Check sheet for the modelled part. Datum: model origin and axes. Units: mm. A direction names the side the tool comes from. Round coordinates to 2 decimals unless told otherwise and drop trailing zeros. Write each loop counter-clockwise with the first axis right and the second up, starting at its lowest first coordinate (ties: lowest second). Pieces come first, ordered by that corner, then holes.
Autodesk Inventor part; units mm, degrees
ref_plane "YZ Plane" through (0, 0, 0) normal (1, 0, 0) x (0, 1, 0)
ref_plane "XZ Plane" through (0, 0, 0) normal (0, 1, 0) x (-1, 0, 0)
ref_plane "XY Plane" through (0, 0, 0) normal (0, 0, 1) x (1, 0, 0)
sketch "Sketch1" plane through (0, 0, 0) normal (0, 1, 0) x (-1, 0, 0)
  line L0 (0, 0) -> (42, 0)
  line L1 (42, 0) -> (42, -42)
  line L2 (42, -42) -> (0, -42)
  line L3 (0, -42) -> (0, 0)
  line L4 (42, -21) -> (42, -5.25)
  line L5 (21, -5.25) -> (36.75, -5.25)
  line L6 (36.75, -5.25) -> (5.25, -5.25)
  line L7 (5.25, -5.25) -> (5.25, -36.75)
  line L8 (5.25, -36.75) -> (36.75, -36.75)
  line L9 (36.75, -36.75) -> (36.75, -5.25)
  circle A0 centre (36.75, -5.25) radius 1.5
  circle A1 centre (36.75, -36.75) radius 1.5
  circle A2 centre (5.25, -36.75) radius 1.5
  circle A3 centre (5.25, -5.25) radius 1.5
  dimension "d6" = 3
  dimension "d7" = 3
  dimension "d8" = 3
  dimension "d9" = 3
extrude "Extrusion1" add sketch "Sketch1" along normal blind 43 contours L0 L1 L2 L3 | L5 A0 L9 A1 L8 A2 L7 A3 L6
sketch "Sketch2" plane through (0, 43, 0) normal (0, 1, 0) x (1, 0, 0)
  circle A0 centre (-21, 21) radius 11
  circle A1 centre (-21, 21) radius 2.5
  point P0 (0, 0)
  dimension "d12" = 22
  dimension "d15" = 5
extrude "Extrusion2" add sketch "Sketch2" along normal blind 3 contours A0 | A1
extrude "Extrusion3" add sketch "Sketch2" along normal blind 25 contours A1
sketch "Sketch3" plane through (0, 0, 0) normal (1, 0, 0) x (0, 0, -1)
  line L0 (42, 0) -> (0, 0)
  line L1 (21, 0) -> (28.5, 0)
  line L2 (28.5, 0) -> (13.5, 0)
  line L3 (13.5, 0) -> (13.5, 12)
  line L4 (13.5, 12) -> (28.5, 12)
  line L5 (28.5, 12) -> (28.5, 0)
  dimension "d18" = 7.5
  dimension "d19" = 15
  dimension "d20" = 12
extrude "Extrusion4" add sketch "Sketch3" along normal blind 8
fillet "Fillet1" radius 4 4 edges at (0, 21.5, 0) (0, 21.5, -42) (-42, 21.5, 0) (-42, 21.5, -42)
properties part number "stepperMotor"
1. Sectioned sample at C-C, the plane x = -36.75. Enter the section's corners in (y, z), plus the area to 3 significant figures.
2. Sectioned sample at A-A, the plane z = -36.75. Enter the section's corners in (x, y).
3. Sectioned sample at B-B, the plane y = 19. Enter the section's corners in (x, z), plus the area to 3 significant figures.
4. Release check for a two-part mould opening along X. For faces 4 (the flat face through (4, 6, -28.5)), 5 (the cylindrical face through (-4.925, 21.199, -35.286)), 6 (the flat face through (-42, 21, -21)), 7 (the cylindrical face through (-35.56, 21.2, -35.84)) record: released by +X, released by -X, zero draft, split by the parting line, or undercut.
5. Sectioned sample at D-D, the plane x = -21. Enter the section's corners in (y, z).
6. Go/stop test with flat-tipped pins: pin 1 (17 mm diameter, centred on y = 16, z = -26.5, fed in from +X); pin 2 (4 mm diameter, centred on x = 3, y = 7, fed in from +Z); pin 3 (2 mm diameter, centred on x = -3.5, z = -32, fed in from +Y); pin 4 (8 mm diameter, centred on y = 24, z = -23.5, fed in from +X). Record where each tip stops, or that it passes through.
7. Scan lines: line 1 along Z through (x, y) = (-5.25, 14); line 2 along X through (y, z) = (8, -6). Record each from-to range of solid material in increasing order.
8. Set-up check for faces 1 (the cylindrical face through (-15.924, 44.479, -30.759)), 2 (the flat face through (4, 12, -21)), 3 (the flat face through (-21, 21, -42)): record each of +Z, -Z, +X, -X, +Y, -Y from which the full face is reachable in a straight line by a thin tool's end or side.
Computed values:
1. outline: (0, -42) - (43, -42) - (43, -38.25) - (0, -38.25) - close; (0, -35.25) - (43, -35.25) - (43, -6.75) - (0, -6.75) - close; (0, -3.75) - (43, -3.75) - (43, 0) - (0, 0) - close
1. area: 1,550 mm2
2. outline: (-42, 0) - (-38.25, 0) - (-38.25, 43) - (-42, 43) - close; (-35.25, 0) - (-6.75, 0) - (-6.75, 43) - (-35.25, 43) - close; (-3.75, 0) - (0, 0) - (0, 43) - (-3.75, 43) - close
3. outline: (-42, -38) arc R4 ccw to (-38, -42) - (-4, -42) arc R4 ccw to (0, -38) - (0, -4) arc R4 ccw to (-4, 0) - (-38, 0) arc R4 ccw to (-42, -4) - close; hole circle Ø3 at (-36.75, -36.75); hole circle Ø3 at (-36.75, -5.25); hole circle Ø3 at (-5.25, -36.75); hole circle Ø3 at (-5.25, -5.25)
3. area: 1,720 mm2
4. face 4: zero draft
4. face 5: undercut
4. face 6: released by -X
4. face 7: undercut
5. outline: (0, -42) - (43, -42) - (43, -32) - (46, -32) - (46, -23.5) - (68, -23.5) - (68, -18.5) - (46, -18.5) - (46, -10) - (43, -10) - (43, 0) - (0, 0) - close
6. pin 1: stops at x = 8
6. pin 2: stops at z = -13.5
6. pin 3: stops at y = 43
6. pin 4: stops at x = 0
7. line 1: z = -42 to -38.25, -35.25 to -6.75, -3.75 to 0
7. line 2: x = -42 to -38.05, -35.45 to -6.55, -3.95 to 0
8. face 1: +Y
8. face 2: +Z, -Z, +X, +Y
8. face 3: -Z, +X, -X, +Y, -Y
